from build123d import *

# Parameters (mm, degrees)
F0_R      = 4
F1_DEPTH  = 3
F2_R      = 6
F3_DEPTH  = 4
F4_R      = 4
F5_DEPTH  = 3.2
F6_R      = 1.8
F7_DEPTH  = 10.201
F8_R      = 2.3
F9_DEPTH  = 3.2
F10_R     = 2.3
F11_DEPTH = 3.2


with BuildPart() as f1:
    # F0 (on Top) → F1 (new body)
    with BuildSketch(Plane.XY):
        Circle(F0_R)
    extrude(amount=F1_DEPTH)

    # F2 (on face) → F3 (join)
    with BuildSketch(Plane.XY.offset(3)):
        Circle(F2_R)
    extrude(amount=F3_DEPTH)

    # F4 (on face) → F5 (join)
    with BuildSketch(Plane.XY.offset(7)):
        Circle(F4_R)
    extrude(amount=F5_DEPTH)

    # F6 (on face) → F7 (cut, through all)
    with BuildSketch(Plane.XY.offset(10.2)):
        Circle(F6_R)
    extrude(amount=-F7_DEPTH, mode=Mode.SUBTRACT)

    # F8 (on face) → F9 (cut)
    with BuildSketch(Plane(origin=(0, 0, 0), x_dir=(1, 0, 0), z_dir=(0, 0, -1))):
        Circle(F8_R)
    extrude(amount=-F9_DEPTH, mode=Mode.SUBTRACT)

    # F10 (on face) → F11 (cut)
    with BuildSketch(Plane.XY.offset(10.2)):
        Circle(F10_R)
    extrude(amount=-F11_DEPTH, mode=Mode.SUBTRACT)


solid = f1.part
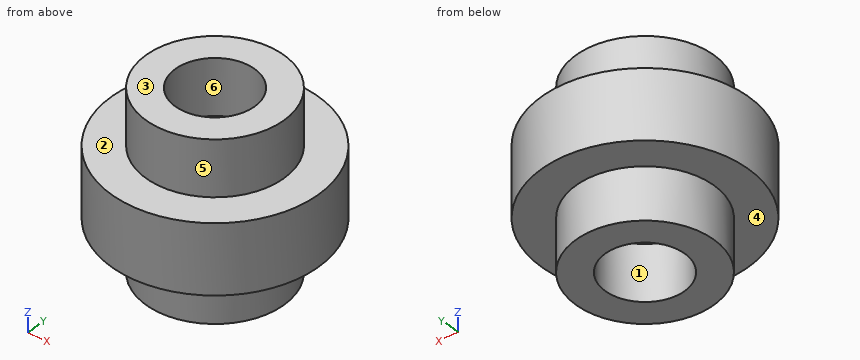
The model under review builds one solid part; all positions refer to its coordinate system, in mm. Face numbers are marked on the shaded views. A direction names the side the tool comes from. Give positions to 0.01 mm unless a question says otherwise; leave off trailing zeros. Loops run counter-clockwise (first coordinate to the right, second up) from the corner with the lowest first, then second, coordinate; pieces in that order, holes last. Notation, with made-up numbers: (44.25, 43.5) -> (64.25, 43.5) arc R13 cw to (64.25, 68.5) -> close; hole circle Ø10 at (-11, 67.25). An arc over 180 degrees is marked (long way). Put each result on its own line as item: value. Start each with the question number.
1. Wall thickness on probe 1 along Y at (x, z) = (0, 4.4); probe 2 along Y at (x, z) = (0, 8.7); probe 3 along Z at (x, y) = (-4, -1.75): over which ranges is each line inside the solid? List them lowest first.
2. Clearance check with flat-ended pins moving along their axes: P1, Ø3, axis at x = 0, y = 0, coming from the +Z side; P2, Ø4.5, axis at x = 0, y = 0, coming from the -Z side; P3, Ø1.5, axis at x = -4.5, y = 2, coming from the -Z side; P4, Ø1.5, axis at x = 2.5, z = 7.5, coming from the +Y side. State where each tip first meets the part, or that it passes through.
3. We need section C-C on y = 3.25. State the section outline as (x, z) points.
4. For the marked faces 1, 2 and 3, list the 3-axis set-ups (+Z, -Z, +X, -X, +Y, -Y) from which the entire face can be reached by the end or side of a thin tool; tool diameter is ignored.
5. Mouldability with a two-part tool opening along Y and no side actions: class the marked faces 4, 5 and 6 as released by +Y, released by -Y, zero draft, split by the parting line, or undercut.
6. We need section D-D on z = 6. State the section outline as (x, y) points, then the cut area to 3 significant figures.
7. We need section A-A on y = 0. State the section outline as (x, z) points.
Determined:
1. probe 1: -6 to -1.8, 1.8 to 6
1. probe 2: -4 to -2.3, 2.3 to 4
1. probe 3: 3 to 7
2. P1: through
2. P2: z = 3.2
2. P3: z = 3
2. P4: y = 5.68
3. outline: (-5.04, 3) -> (-2.33, 3) -> (-2.33, 0) -> (2.33, 0) -> (2.33, 3) -> (5.04, 3) -> (5.04, 7) -> (2.33, 7) -> (2.33, 10.2) -> (-2.33, 10.2) -> (-2.33, 7) -> (-5.04, 7) -> close
4. face 1: -Z
4. face 2: +Z
4. face 3: +Z, +X, -X, +Y, -Y
5. face 4: zero draft
5. face 5: split by the parting line
5. face 6: undercut
6. outline: circle Ø12 at (0, 0); hole circle Ø3.6 at (0, 0)
6. area: 103 mm^2
7. outline: (-6, 3) -> (-4, 3) -> (-4, 0) -> (-2.3, 0) -> (-2.3, 3.2) -> (-1.8, 3.2) -> (-1.8, 7) -> (-2.3, 7) -> (-2.3, 10.2) -> (-4, 10.2) -> (-4, 7) -> (-6, 7) -> close; (1.8, 3.2) -> (2.3, 3.2) -> (2.3, 0) -> (4, 0) -> (4, 3) -> (6, 3) -> (6, 7) -> (4, 7) -> (4, 10.2) -> (2.3, 10.2) -> (2.3, 7) -> (1.8, 7) -> close
